```python
from build123d import *

# Parameters (mm, degrees)
SKETCH1_W           = 88
SKETCH1_H           = 50
BOSS_EXTRUDE1_DEPTH = 18
BOSS_EXTRUDE2_DEPTH = 38
SKETCH5_W           = 74.105007355
SKETCH5_H           = 76.56039949
CUT_EXTRUDE1_DEPTH  = 38


with BuildPart() as part:
    # Sketch1 → Boss-Extrude1 (new body)
    with BuildSketch(Plane(origin=(0, 0, 0), x_dir=(1, 0, 0), z_dir=(0, 1, 0))):
        Rectangle(SKETCH1_W, SKETCH1_H)
    extrude(amount=BOSS_EXTRUDE1_DEPTH)

    # Sketch2 → Boss-Extrude2 (add)
    with BuildSketch(Plane(origin=(0, 18, 0), x_dir=(1, 0, 0), z_dir=(0, 1, 0))):
        Polygon((-44, 3), (-6, 3), (-6, -24.990461848), (6, -24.990461848), (6, 3), (44, 3), (44, 15), (6, 15), (6, 25), (-6, 25), (-6, 15), (-44, 15), align=None)
    extrude(amount=BOSS_EXTRUDE2_DEPTH)

    # Sketch5 → Cut-Extrude1 (cut)
    with BuildSketch(Plane(origin=(22.123893805, 22.123893805, 24.778761062), x_dir=(-0.8323002445923469, 0.36918924973045525, 0.4134919596981098), z_dir=(-0.5543250876981122, -0.5543250876981184, -0.6208440982218917))):
        with Locations((7.332126574, 18.101961107)):
            Rectangle(SKETCH5_W, SKETCH5_H)
    extrude(amount=-CUT_EXTRUDE1_DEPTH, mode=Mode.SUBTRACT)


solid = part.part
```
Part model, mm, in its own coordinate system. A direction names the side the tool comes from. Round coordinates to 2 decimals unless told otherwise and drop trailing zeros. Loops run counter-clockwise (first coordinate to the right, second up) from the corner with the lowest first, then second, coordinate; pieces in that order, holes last.
Item 1: 3-axis set-ups, long thin cutter, end or side, ignore diameter. For faces 1 (the face through (-25, 37, -3)), 2 (the face through (-10, 18, 11)), 3 (the face through (21, 33, -3)): which of +Z, -Z, +X, -X, +Y, -Y reach the whole face in a straight line?
Item 2: Cut at D-D, the plane z = -10.5. Give the cut face in (x, y), then the cut area to 3 significant figures.
Item 3: Cut at C-C, the plane z = -17. Give the cut face in (x, y), then the cut area to 3 significant figures.
Item 4: Drill centre lines: line 1 (Y direction, x = 10, z = 7); line 2 (Z direction, x = 22, y = 34); line 3 (X direction, y = 44.5, z = 11). Where is each one in solid material? Low to high.
Item 5: Drop flat-ended pins along their axis: P1, Ø11, axis at y = 43.5, z = -22.5, coming from the -X side; P2, Ø3, axis at y = 40.5, z = -20, coming from the +X side; P3, Ø6, axis at x = 2.5, y = 26, coming from the +Z side. Give the stop position or say it passes through.
Item 6: Cut at A-A, the plane y = 28. Give the cut face in (x, z).
Item 7: Cut at B-B, the plane x = -33.5. Give the cut face in (y, z).
A:
1. face 1: +Z, -X, +Y
1. face 2: +Z, +Y
1. face 3: +Z, +X, +Y
2. outline: (-44, 0) - (44, 0) - (44, 39.76) - (27.76, 56) - (-44, 56) - close
2. area: 4,800 mm2
3. outline: (-44, 0) - (44, 0) - (44, 18) - (6, 18) - (6, 56) - (-6, 56) - (-6, 18) - (-44, 18) - close
3. area: 2,040 mm2
4. line 1: y = 0 to 18
4. line 2: z = -15 to -3
4. line 3: x = -6 to 6
5. P1: stops at x = -6
5. P2: stops at x = 6
5. P3: stops at z = 24.99
6. outline: (-44, -15) - (-6, -15) - (-6, -25) - (6, -25) - (6, -15) - (44, -15) - (44, -3) - (6, -3) - (6, 24.99) - (-6, 24.99) - (-6, -3) - (-44, -3) - close
7. outline: (0, -25) - (18, -25) - (18, -15) - (56, -15) - (56, -3) - (18, -3) - (18, 25) - (0, 25) - close
